from build123d import *

# Parameters (mm, degrees)
SKETCH1_R           = 12.7
SKETCH1_R_2         = 10.7
SKETCH1_R_3         = 0.8
SKETCH1_R_4         = 1.5
SKETCH1_R_5         = 3.6
BOSS_EXTRUDE1_DEPTH = 3
BOSS_EXTRUDE2_START = -3
SKETCH1_3_R         = 12.7
SKETCH1_3_R_2       = 10.7
BOSS_EXTRUDE2_DEPTH = 3
SKETCH2_R           = 4.5
CUT_EXTRUDE1_DEPTH  = 10


with BuildPart() as part:
    # Sketch1 → Boss-Extrude1 (new body)
    # profile 1 of 4: a face of its own
    with BuildSketch(Plane(origin=(0, 0, 0), x_dir=(1, 0, 0), z_dir=(0, 1, 0))):
        Circle(SKETCH1_R)
        Circle(SKETCH1_R_2, mode=Mode.SUBTRACT)
    # profile 2 of 4: a face of its own
    with BuildSketch(Plane(origin=(0, 0, 0), x_dir=(1, 0, 0), z_dir=(0, 1, 0))):
        Circle(SKETCH1_R_2)
        with Locations(Location((0, -7.2, 0), (0, 0, 270))):
            Circle(SKETCH1_R_3, mode=Mode.SUBTRACT)
        with Locations(Location((7.2, 0, 0), (0, 0, 270))):
            Circle(SKETCH1_R_3, mode=Mode.SUBTRACT)
        with Locations(Location((0, 7.2, 0), (0, 0, 270))):
            Circle(SKETCH1_R_3, mode=Mode.SUBTRACT)
        with Locations(Location((-7.2, 0, 0), (0, 0, 270))):
            Circle(SKETCH1_R_3, mode=Mode.SUBTRACT)
        with Locations(Location((0, 0, 0), (0, 0, 270))):
            Circle(SKETCH1_R_4, mode=Mode.SUBTRACT)
    # profile 3 of 4: a face of its own
    with BuildSketch(Plane(origin=(0, 0, 0), x_dir=(1, 0, 0), z_dir=(0, 1, 0))):
        with BuildLine():
            ThreePointArc((35, -3.6), (31.4, 0), (35, 3.6))
            Line((35, 3.6), (5.526066251, 11.434709956))
            ThreePointArc((5.526066251, 11.434709956), (10.758044464, 6.749405848), (12.7, 0))
            ThreePointArc((12.7, 0), (10.758044464, -6.749405848), (5.526066251, -11.434709956))
            Line((5.526066251, -11.434709956), (35, -3.6))
        make_face()
    # profile 4 of 4: a face of its own
    with BuildSketch(Plane(origin=(0, 0, 0), x_dir=(1, 0, 0), z_dir=(0, 1, 0))):
        with Locations((35, 0)):
            Circle(SKETCH1_R_5)
        with Locations(Location((35, 0, 0), (0, 0, 270))):
            Circle(SKETCH1_R_4, mode=Mode.SUBTRACT)
    extrude(amount=BOSS_EXTRUDE1_DEPTH)

    # Sketch1_3 → Boss-Extrude2 (add)
    with BuildSketch(Plane(origin=(0, 0, 0), x_dir=(1, 0, 0), z_dir=(0, 1, 0)).offset(BOSS_EXTRUDE2_START)):
        with Locations(Location((0, 0, 0), (0, 0, 64.206858382))):
            Circle(SKETCH1_3_R)
        with Locations(Location((0, 0, 0), (0, 0, 270))):
            Circle(SKETCH1_3_R_2, mode=Mode.SUBTRACT)
    extrude(amount=BOSS_EXTRUDE2_DEPTH)

    # Sketch2 → Cut-Extrude1 (cut)
    with BuildSketch(Plane.XZ):
        with Locations(Location((0, 0, 0), (0, 0, 270))):
            Circle(SKETCH2_R)
    extrude(amount=-CUT_EXTRUDE1_DEPTH, mode=Mode.SUBTRACT)


solid = part.part
The listing builds one solid part. Answer for the finished solid, in the listing's coordinates (mm). A direction names the side the tool comes from. Coordinates: 2 decimals unless noted, no trailing zeros. Write each loop counter-clockwise with the first axis right and the second up, starting at its lowest first coordinate (ties: lowest second). Pieces come first, ordered by that corner, then holes. Notation, with made-up numbers: (62, 32) - (112, 32) arc R13 cw to (112, 45) - close; hole circle Ø5 at (-32, 19). An arc over 180 degrees is marked (long way). Answer as CSV lines item,"result".
1. Given P1, Ø1.5, axis at x = 8, y = -1.5, coming from the +Z side; P2, Ø2, axis at x = 23.5, y = 0.5, coming from the +Z side; P3, Ø1.8, axis at x = -7.2, z = 0, coming from the -Y side; P4, Ø1.4, axis at x = 0, z = -7.2, coming from the -Y side, each flat-ended and moving along its own axis, determine where each tip first touches the part or whether it passes through.
Computed values:
P1,"stops at z = 10.43"
P2,"stops at z = 6.92"
P3,"stops at y = 0"
P4,"passes through"
2. Find section A-A (z = 0). Give the vertices of the cut face in (x, y).
Computed values:
outline,"(-12.7, -3) - (-10.7, -3) - (-10.7, 0) - (-8, 0) - (-8, 3) - (-12.7, 3) - close; (-6.4, 0) - (-4.5, 0) - (-4.5, 3) - (-6.4, 3) - close; (4.5, 0) - (6.4, 0) - (6.4, 3) - (4.5, 3) - close; (8, 0) - (10.7, 0) - (10.7, -3) - (12.7, -3) - (12.7, 0) - (33.5, 0) - (33.5, 3) - (8, 3) - close; (36.5, 0) - (38.6, 0) - (38.6, 3) - (36.5, 3) - close"
3. Find section D-D (x = -7.2). Give the vertices of the cut face in (y, z).
Computed values:
outline,"(-3, -10.46) - (3, -10.46) - (3, -0.8) - (0, -0.8) - (0, -7.92) - (-3, -7.92) - close; (-3, 7.92) - (0, 7.92) - (0, 0.8) - (3, 0.8) - (3, 10.46) - (-3, 10.46) - close"
4. Find section B-B (x = 0). Give the vertices of the cut face in (y, z).
Computed values:
outline,"(-3, -12.7) - (3, -12.7) - (3, -8) - (0, -8) - (0, -10.7) - (-3, -10.7) - close; (-3, 10.7) - (0, 10.7) - (0, 8) - (3, 8) - (3, 12.7) - (-3, 12.7) - close; (0, -6.4) - (3, -6.4) - (3, -4.5) - (0, -4.5) - close; (0, 4.5) - (3, 4.5) - (3, 6.4) - (0, 6.4) - close"
5. A tool of negligible diameter and unlimited length cuts with its end or side. For faces 5 (the cylindrical face through (-10.446, -1.521, -2.32)), 6 (the cylindrical face through (-6.407, 1.479, -0.104)), from which of +Z, -Z, +X, -X, +Y, -Y can it reach the whole face along a straight path? Write none if from no direction.
Computed values:
face 5,"-Y"
face 6,"+Y, -Y"
6. Straight lines are drawn through the part: line 1 (X direction, y = 1.9, z = 0); line 2 (Y direction, x = 7.5, z = 10.75); line 3 (X direction, y = -0.95, z = -2.5). For each, find the intervals that lie inside material, in ascending order. Write a range as [from, to].
Computed values:
line 1,"x = [-12.7, -8], [-6.4, -4.5], [4.5, 6.4], [8, 33.5], [36.5, 38.6]"
line 2,"y = [0, 3]"
line 3,"x = [-12.45, -10.4], [10.4, 12.45]"
7. Find section C-C (y = 2.1). Give the vertices of the cut face in (x, z).
Computed values:
outline,"(5.53, -11.43) - (35, -3.6) arc R3.6 ccw to (35, 3.6) - (5.53, 11.43) arc R12.7 ccw (long way) to start; hole circle Ø1.6 at (-7.2, 0); hole circle Ø9 at (0, 0); hole circle Ø1.6 at (0, -7.2); hole circle Ø1.6 at (0, 7.2); hole circle Ø1.6 at (7.2, 0); hole circle Ø3 at (35, 0)"
8. Determine the mould class of faces 1 (the cylindrical face through (33.536, 1.479, -0.325)), 2 (the flat face through (22, 0, 0)), 3 (the cylindrical face through (1.352, 1.479, -4.292)), 4 (the cylindrical face through (38.6, 1.5, 0.1)) for opening direction Z: +Z half, -Z half, draft (parallel to the pull), parting line (faces both ways), or undercut.
Computed values:
face 1,"undercut"
face 2,"draft"
face 3,"undercut"
face 4,"parting line"
